Geometry check sheet. Reference: drawing and pictorial views, mm from the part's lowest x, y, z. A direction names the side the tool comes from. Coordinates: 2 decimals unless noted, no trailing zeros. Loops run counter-clockwise (first coordinate to the right, second up) from the corner with the lowest first, then second, coordinate; pieces in that order, holes last.
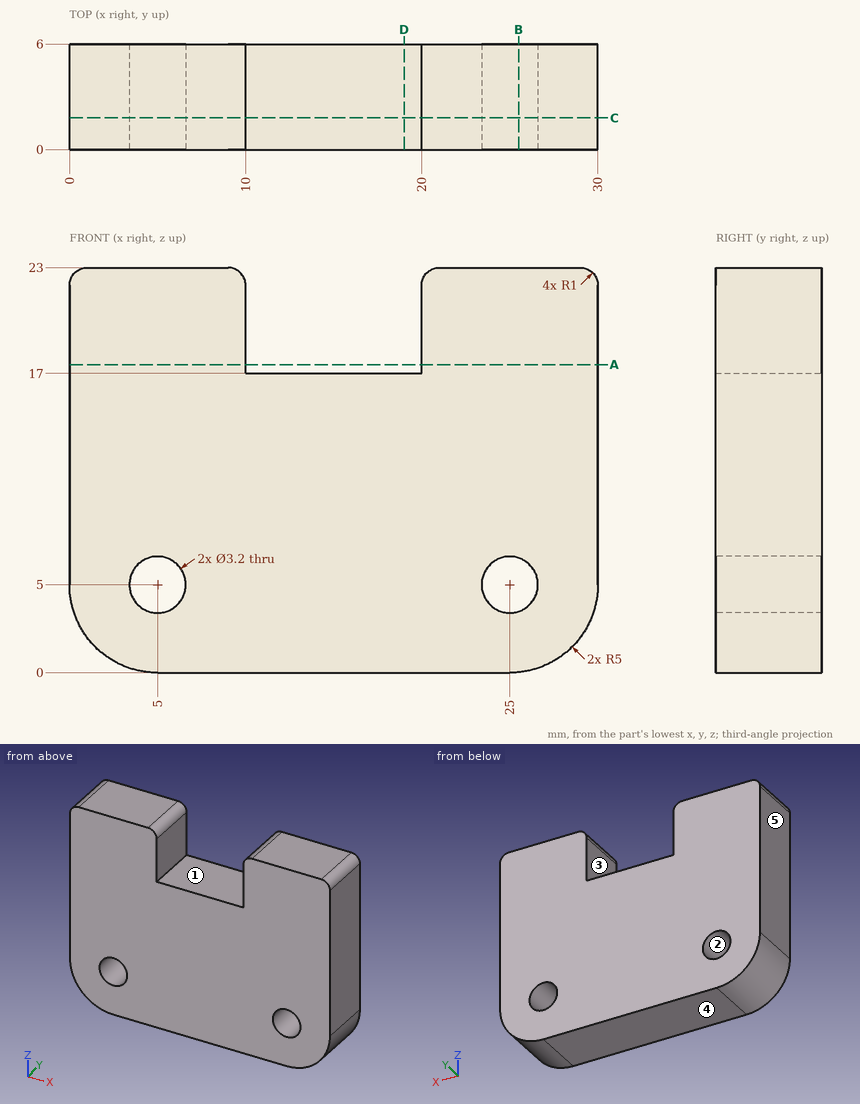
1) Access from +Z, -Z, +X, -X, +Y, -Y to the whole of each face (thin tool, end or side, straight path). Record for the marked faces 1 and 2.
Data:
face 1: +Z, +Y, -Y
face 2: +Y, -Y
2) Section check A-A on z = 17.5. Record the cut outline in (x, y), and give its area (3 significant figures).
Data:
outline: (0, 0) - (10, 0) - (10, 6) - (0, 6) - close; (20, 0) - (30, 0) - (30, 6) - (20, 6) - close
area: 120 mm2
3) Section check C-C on y = 1.8. Record the cut outline in (x, z), and give its area (3 significant figures).
Data:
outline: (0, 5) arc R5 ccw to (5, 0) - (25, 0) arc R5 ccw to (30, 5) - (30, 22) arc R1 ccw to (29, 23) - (21, 23) arc R1 ccw to (20, 22) - (20, 17) - (10, 17) - (10, 22) arc R1 ccw to (9, 23) - (1, 23) arc R1 ccw to (0, 22) - close; hole circle Ø3.2 at (5, 5); hole circle Ø3.2 at (25, 5)
area: 602 mm2
4) Mould release check, pull along X, two halves, no side actions. Record for the marked faces 3, 4 and 5: +X half, -X half, draft (parallel to the pull), parting line (faces both ways), or undercut.
Data:
face 3: undercut
face 4: draft
face 5: -X half
5) Material ranges on probe 1 along X at (y, z) = (1.8, 5); probe 2 along X at (y, z) = (3.65, 19.25); probe 3 along Z at (x, y) = (25, 2.95), recorded low to high.
Data:
probe 1: x = 0 to 3.4, 6.6 to 23.4, 26.6 to 30
probe 2: x = 0 to 10, 20 to 30
probe 3: z = 0 to 3.4, 6.6 to 23
6) Depth check by flat-ended pin: pin 1 (1.8 mm diameter, centred on x = 16, y = 3.5, fed in from +Z). Enter the tip coordinate at first touch or a pass-through.
Data:
pin 1: stops at z = 17
7) Section check D-D on x = 19. Record the cut outline in (y, z), and give its area (3 significant figures).
Data:
outline: (0, 0) - (6, 0) - (6, 17) - (0, 17) - close
area: 102 mm2
8) Section check B-B on x = 25.5. Record the cut outline in (y, z), and give its area (3 significant figures).
Data:
outline: (0, 0.03) - (6, 0.03) - (6, 3.48) - (0, 3.48) - close; (0, 6.52) - (6, 6.52) - (6, 23) - (0, 23) - close
area: 120 mm2
